```python
from build123d import *

# Parameters (mm, degrees)
SKETCH10_W          = 50.2
SKETCH10_H          = 5
BOSS_EXTRUDE5_DEPTH = 27.2
SKETCH15_W          = 45.2
SKETCH15_H          = 25.2
CUT_EXTRUDE7_DEPTH  = 48.330596764
SKETCH16_W          = 1.5
SKETCH16_H          = 5
CUT_EXTRUDE8_DEPTH  = 25.2
SKETCH17_W          = 1.5
SKETCH17_H          = 5
CUT_EXTRUDE9_DEPTH  = 25.2
SKETCH19_W          = 2
SKETCH19_H          = 5
BOSS_EXTRUDE6_DEPTH = 2.5
SKETCH20_W          = 2
SKETCH20_H          = 5
BOSS_EXTRUDE7_DEPTH = 2.5
SKETCH21_R          = 1.5
CUT_EXTRUDE10_DEPTH = 2.5
FILLET4_R           = 0.1
SKETCH22_R          = 1.5
CUT_EXTRUDE11_DEPTH = 2.5
FILLET5_R           = 0.1


with BuildPart() as part:
    # Sketch10 → Boss-Extrude5 (new body)
    with BuildSketch(Plane.XY):
        with Locations((-13.310225071, -72.576377738)):
            Rectangle(SKETCH10_W, SKETCH10_H)
    extrude(amount=BOSS_EXTRUDE5_DEPTH)

    # Sketch15 → Cut-Extrude7 (cut, through all)
    with BuildSketch(Plane(origin=(0, -75.076377738, 0), x_dir=(-1, 0, 0), z_dir=(0, -1, 0))):
        with Locations((13.310225071, -12.6)):
            Rectangle(SKETCH15_W, SKETCH15_H)
    extrude(amount=-CUT_EXTRUDE7_DEPTH, mode=Mode.SUBTRACT)

    # Sketch16 → Cut-Extrude8 (cut)
    with BuildSketch(Plane.XY.offset(27.2)):
        with Locations((-37.660225071, -72.576377738)):
            Rectangle(SKETCH16_W, SKETCH16_H)
    extrude(amount=-CUT_EXTRUDE8_DEPTH, mode=Mode.SUBTRACT)

    # Sketch17 → Cut-Extrude9 (cut)
    with BuildSketch(Plane.XY.offset(27.2)):
        with Locations((11.039774929, -72.576377738)):
            Rectangle(SKETCH17_W, SKETCH17_H)
    extrude(amount=-CUT_EXTRUDE9_DEPTH, mode=Mode.SUBTRACT)

    # Sketch19 → Boss-Extrude6 (add)
    with BuildSketch(Plane.ZY.offset(38.410225071)):
        with Locations((1, -72.576377738)):
            Rectangle(SKETCH19_W, SKETCH19_H)
    extrude(amount=BOSS_EXTRUDE6_DEPTH)

    # Sketch20 → Boss-Extrude7 (add)
    with BuildSketch(Plane(origin=(11.789774929, 0, 0), x_dir=(0, 0, -1), z_dir=(1, 0, 0))):
        with Locations((-1, -72.576377738)):
            Rectangle(SKETCH20_W, SKETCH20_H)
    extrude(amount=BOSS_EXTRUDE7_DEPTH)

    # Sketch21 → Cut-Extrude10 (cut)
    with BuildSketch(Plane.XY.offset(2)):
        with Locations((-38.910225071, -72.576377738)):
            Circle(SKETCH21_R)
    extrude(amount=-CUT_EXTRUDE10_DEPTH, mode=Mode.SUBTRACT)

    # Fillet4
    fillet4_edges = [part.edges().sort_by_distance(p)[0] for p in [
        (-40.410225071, -72.576377738, 2),
    ]]
    fillet(fillet4_edges, radius=FILLET4_R)

    # Sketch22 → Cut-Extrude11 (cut)
    with BuildSketch(Plane.XY.offset(2)):
        with Locations((12.289774929, -72.576377738)):
            Circle(SKETCH22_R)
    extrude(amount=-CUT_EXTRUDE11_DEPTH, mode=Mode.SUBTRACT)

    # Fillet5
    fillet5_edges = [part.edges().sort_by_distance(p)[0] for p in [
        (10.789774929, -72.576377738, 2),
    ]]
    fillet(fillet5_edges, radius=FILLET5_R)


solid = part.part
```
Geometry check sheet. Reference: the model listing, model coordinates, mm. A direction names the side the tool comes from. Round coordinates to 2 decimals unless told otherwise and drop trailing zeros. Loops run counter-clockwise (first coordinate to the right, second up) from the corner with the lowest first, then second, coordinate; pieces in that order, holes last. Notation, with made-up numbers: M -10.75,-27.75 L 15.25,-27.75 A16 cw 15.25,-19.75 Z; hole C 25.25,46.25 d7. An arc over 180 degrees is marked long. Return JSON: item names as keys, results as strings. Group by question number.
(1) Section check A-A, the plane z = 2.75. Enter the section's corners in (x, y), and give its area (4 significant figures).
(2) Section check C-C, the plane x = -10. Enter the section's corners in (y, z).
(3) Set-up check for faces 4 (the face through (-38, -71, 2)), 5 (the face through (12.7, -74.3, 2)), 6 (the face through (-13, -73, 25.2)): record each of +Z, -Z, +X, -X, +Y, -Y from which the full face is reachable in a straight line by a thin tool's end or side.
(4) Section check B-B, the plane y = -73.15. Give the number of separate pieces and of enclosed holes in the cut face, and give its area (3 significant figures).
(5) Scan lines: line 1 along X through (y, z) = (-73.5, 21.75); line 2 along Z through (x, y) = (-19, -70.6). Record each from-to range of solid material in increasing order. Write a range as [from, to].
(6) Mould release check, pull along X, two halves, no side actions. Record for faces 1 (the face through (9.29, -73, 13)), 2 (the face through (10.29, -73, 15)), 3 (the face through (-20, -70.076, 26)): pulls with the +X half, pulls with the -X half, needs draft (parallel to the pull), parting line crosses it, or undercut.
(7) Go/stop test with flat-tipped pins: pin 1 (3 mm diameter, centred on x = -39.5, y = -74, fed in from +Z); pin 2 (2.5 mm diameter, centred on y = -73, z = 16, fed in from -X); pin 3 (2.5 mm diameter, centred on y = -72, z = 20.5, fed in from +X); pin 4 (1.8 mm diameter, centred on x = 12.29, y = -72.58, fed in from -Z) (1 decimal). Record where each tip stops, or that it passes through.
Data:
{
 "1": {"outline": "M -36.91,-75.08 L -35.91,-75.08 L -35.91,-70.08 L -36.91,-70.08 Z; M 9.29,-75.08 L 10.29,-75.08 L 10.29,-70.08 L 9.29,-70.08 Z", "area": "10.00 mm²"},
 "2": {"outline": "M -75.08,25.2 L -70.08,25.2 L -70.08,27.2 L -75.08,27.2 Z"},
 "3": {"face 4": "+Z, -X, +Y, -Y", "face 5": "+Z, +X, +Y, -Y", "face 6": "-Z, +Y, -Y"},
 "4": {"separate pieces": "3", "enclosed holes": "0", "area": "150 mm²"},
 "5": {"line 1": "[-36.91, -35.91], [9.29, 10.29]", "line 2": "[25.2, 27.2]"},
 "6": {"face 1": "undercut", "face 2": "pulls with the +X half", "face 3": "needs draft"},
 "7": {"pin 1": "z = 2", "pin 2": "x = -36.91", "pin 3": "x = 10.29", "pin 4": "through"}
}
